The drawing under review shows one solid part. Ordinate dimensions are in mm from its lowest x, y, z. Coordinates: 2 decimals unless noted, no trailing zeros. Write each loop counter-clockwise with the first axis right and the second up, starting at its lowest first coordinate (ties: lowest second). Pieces come first, ordered by that corner, then holes. Notation, with made-up numbers: (-1.5, -17) - (10.5, -17) arc R30 cw to (10.5, 9) - close; hole circle Ø2 at (-14.5, -19). An arc over 180 degrees is marked (long way). Put each result on its own line as item: value. Start each with the question number.
Item 1: To check wall thickness, follow L1, parallel to X at y = 22, z = 3.5; L2, parallel to Z at x = 34.5, y = 33; L3, parallel to Y at x = 7.5, z = 12.5. State the ranges of each line that lie inside material, in increasing order. Write a range as [from, to].
Item 2: For pin 1 (1 mm diameter, centred on x = 40, y = 34, fed in from +Z); pin 2 (2.5 mm diameter, centred on y = 30, z = 13, fed in from -X); pin 3 (1.5 mm diameter, centred on y = 17, z = 13.5, fed in from +X), all flat-tipped, find the tip position at first contact; note any pin that passes through.
Item 3: Consider section B-B on x = 17.5. Give the boundary of the cut face in (y, z), then the cut area to 3 significant figures.
Item 4: Consider section A-A on z = 3.5. Give the boundary of the cut face in (x, y).
Item 5: Mouldability with a two-part tool opening along X and no side actions: class the marked faces 1, 2 and 3 as pulls with the +X half, pulls with the -X half, needs draft (parallel to the pull), parting line crosses it, or undercut.
Item 6: Consider section D-D on z = 12.75. Give the boundary of the cut face in (x, y).
Item 7: Consider section C-C on y = 23. Give the boundary of the cut face in (x, z).
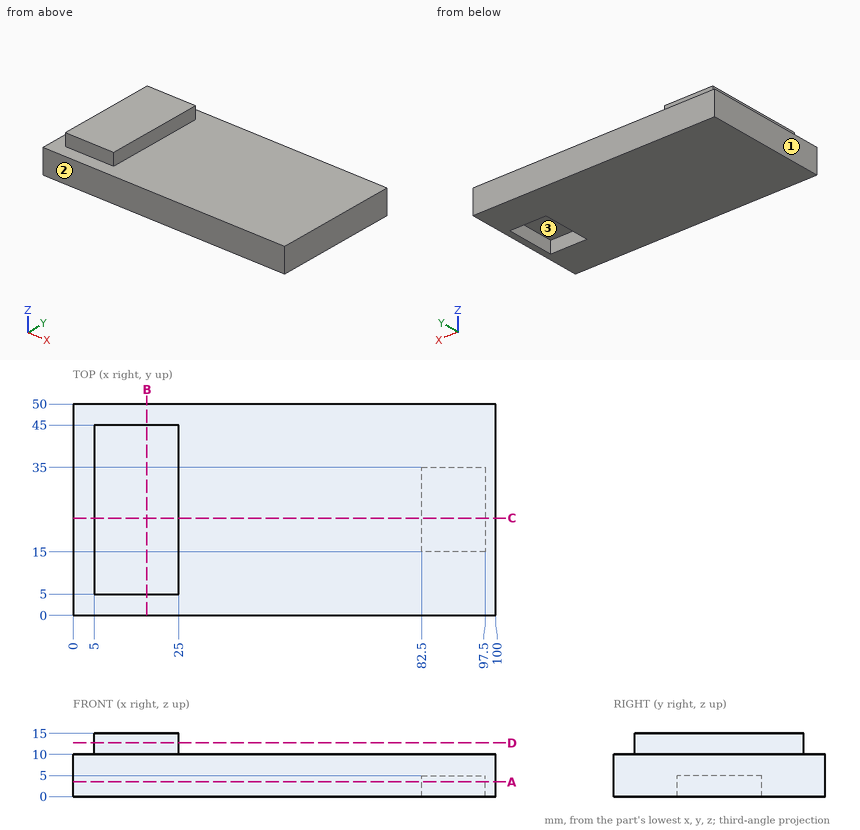
Report:
1. L1: [0, 82.5], [97.5, 100]
1. L2: [0, 10]
1. L3: [5, 45]
2. pin 1: z = 10
2. pin 2: x = 5
2. pin 3: x = 25
3. outline: (0, 0) - (50, 0) - (50, 10) - (45, 10) - (45, 15) - (5, 15) - (5, 10) - (0, 10) - close
3. area: 700 mm²
4. outline: (0, 0) - (100, 0) - (100, 50) - (0, 50) - close; hole (82.5, 15) - (97.5, 15) - (97.5, 35) - (82.5, 35) - close
5. face 1: pulls with the -X half
5. face 2: needs draft
5. face 3: undercut
6. outline: (5, 5) - (25, 5) - (25, 45) - (5, 45) - close
7. outline: (0, 0) - (82.5, 0) - (82.5, 5) - (97.5, 5) - (97.5, 0) - (100, 0) - (100, 10) - (25, 10) - (25, 15) - (5, 15) - (5, 10) - (0, 10) - close
